Geometry check sheet. Reference: the model listing, model coordinates, mm. A direction names the side the tool comes from. Round coordinates to 2 decimals unless told otherwise and drop trailing zeros. Loops run counter-clockwise (first coordinate to the right, second up) from the corner with the lowest first, then second, coordinate; pieces in that order, holes last. Notation, with made-up numbers: M 34.5,89 L 45.5,89 A23 ccw 45.5,116 Z; hole C 76.25,30.25 d1. An arc over 180 degrees is marked long. Use one line per item in the form item = value. Start each with the question number.
1. Go/stop test with flat-tipped pins: pin 1 (22 mm diameter, centred on x = -24.5, y = -12, fed in from -Z); pin 2 (9 mm diameter, centred on x = -11, z = 16, fed in from -Y); pin 3 (22 mm diameter, centred on x = -19.5, z = 48, fed in from +Y); pin 4 (2 mm diameter, centred on x = -32.5, z = 39.5, fed in from +Y). Record where each tip stops, or that it passes through.
2. Cross-section at A-A (y = -8). Record the boundary of the cut face in (x, z), then the cut area to 3 significant figures.
3. Cross-section at D-D (y = 4.5). Record the boundary of the cut face in (x, z).
4. Draft check along Y on faces 1 (the flat face through (-20, -6, 51.505)), 2 (the flat face through (-20, -24.08, 57)), 3 (the flat face through (-20, 30, 15)). Enter one of: pulls with the +Y half, pulls with the -Y half, needs draft (parallel to the pull), parting line crosses it, or undercut.
5. Cross-section at B-B (x = -24). Record the boundary of the cut face in (y, z), then the cut area to 3 significant figures.
6. Cross-section at C-C (y = 26). Record the boundary of the cut face in (x, z).
7. Material ranges on line 1 (Z direction, x = -14.5, y = -4); line 2 (Z direction, x = -16.5, y = 10.5); line 3 (Y direction, x = -27.5, z = 23.5), recorded low to high.
8. Set-up check for faces 4 (the flat face through (-10, 2, 43)), 5 (the flat face through (-20, 27.158, 46)), 6 (the flat face through (-20, -12, 30)), 7 (the flat face through (-20, 13.191, 48)), 8 (the flat face through (-30, 2, 43)): record each of +Z, -Z, +X, -X, +Y, -Y from which the full face is reachable in a straight line by a thin tool's end or side.
```python
from build123d import *

# Parameters (mm, degrees)
ESQUISSE1_W        = 40
ESQUISSE1_H        = 30
BOSS_EXTRU_1_DEPTH = 30
BOSS_EXTRU_2_START = -10
BOSS_EXTRU_2_DEPTH = 20


with BuildPart() as part:
    # Esquisse1 → Boss.-Extru.1 (new body)
    with BuildSketch(Plane.XY):
        with Locations((-20, 15)):
            Rectangle(ESQUISSE1_W, ESQUISSE1_H)
    extrude(amount=BOSS_EXTRU_1_DEPTH)

    # Esquisse2 → Boss.-Extru.2 (add)
    with BuildSketch(Plane.ZY.offset(40).offset(BOSS_EXTRU_2_START)):
        Polygon((30, 27.158170339), (63.156193336, 27.158170339), (63.156193336, -24.079833233), (51.504613428, -24.079833233), (51.504613428, 13.190748461), (43.833386904, 13.190748461), (43.833386904, -24.079833233), (30, -24.079833233), align=None)
    extrude(amount=-BOSS_EXTRU_2_DEPTH)


solid = part.part
```
Reported:
q1.pin_1 = 30
q1.pin_2 = 0
q1.pin_3 = 27.16
q1.pin_4 = through
q2.outline = M -30,30 L -10,30 L -10,43.83 L -30,43.83 Z; M -30,51.5 L -10,51.5 L -10,63.16 L -30,63.16 Z
q2.area = 510 mm²
q3.outline = M -40,0 L 0,0 L 0,30 L -10,30 L -10,43.83 L -30,43.83 L -30,30 L -40,30 Z; M -30,51.5 L -10,51.5 L -10,63.16 L -30,63.16 Z
q4.face_1 = needs draft
q4.face_2 = pulls with the -Y half
q4.face_3 = pulls with the +Y half
q5.outline = M -24.08,30 L 0,30 L 0,0 L 30,0 L 30,30 L 27.16,30 L 27.16,63.16 L -24.08,63.16 L -24.08,51.5 L 13.19,51.5 L 13.19,43.83 L -24.08,43.83 Z
q5.area = 2,310 mm²
q6.outline = M -40,0 L 0,0 L 0,30 L -10,30 L -10,63.16 L -30,63.16 L -30,30 L -40,30 Z
q7.line_1 = 30 to 43.83, 51.5 to 63.16
q7.line_2 = 0 to 43.83, 51.5 to 63.16
q7.line_3 = 0 to 30
q8.face_4 = +Z, +X, +Y, -Y
q8.face_5 = +Z, +X, -X, +Y
q8.face_6 = -Z, +X, -X, -Y
q8.face_7 = +X, -X, -Y
q8.face_8 = +Z, -X, +Y, -Y
